The drawing under review shows one solid part. Ordinate dimensions are in mm from its lowest x, y, z. A direction names the side the tool comes from. Give positions to 0.01 mm unless a question says otherwise; leave off trailing zeros. Order: outer loops, then holes, each group sorted by start corner. A loop starts at its lowest first (then second) coordinate and runs counter-clockwise, first axis right, second up. Notation, with made-up numbers: (82, -37.5) -> (116, -37.5) arc R26 cw to (116, -6.5) -> close; hole circle Ø6 at (74.5, -23.75). An arc over 180 degrees is marked (long way). One line per item, written item: value. Start each with the question number.
1) Consider section A-A (x = 29.5). State the section outline as (y, z) points.
2) Consider section C-C (y = 54.5). State the section outline as (x, z) points, plus the area to 3 significant figures.
3) Wall thickness on line 1 along Y through (x, z) = (18.5, 11.75); line 2 along X through (y, z) = (67, 18.5): over which ranges is each line inside the solid? List them lowest first. Write a range as from..to.
4) Consider section B-B (z = 13). State the section outline as (x, y) points, plus the area to 3 significant figures.
5) The part is to be moulded in two halves that separate along X. For the marked faces 1, 2, 3 and 4, say which applies: released by +X, released by -X, zero draft, split by the parting line, or undercut.
6) For pin 1 (3 mm diameter, centred on y = 26.5, z = 14.5, fed in from -X), flat-tipped, find the tip position at first contact; note if it passes through.
7) Tool access review of the marked faces 5 and 6: name each direction out of +Z, -Z, +X, -X, +Y, -Y from which nothing blocks a thin tool from reaching the whole face with its end or side.
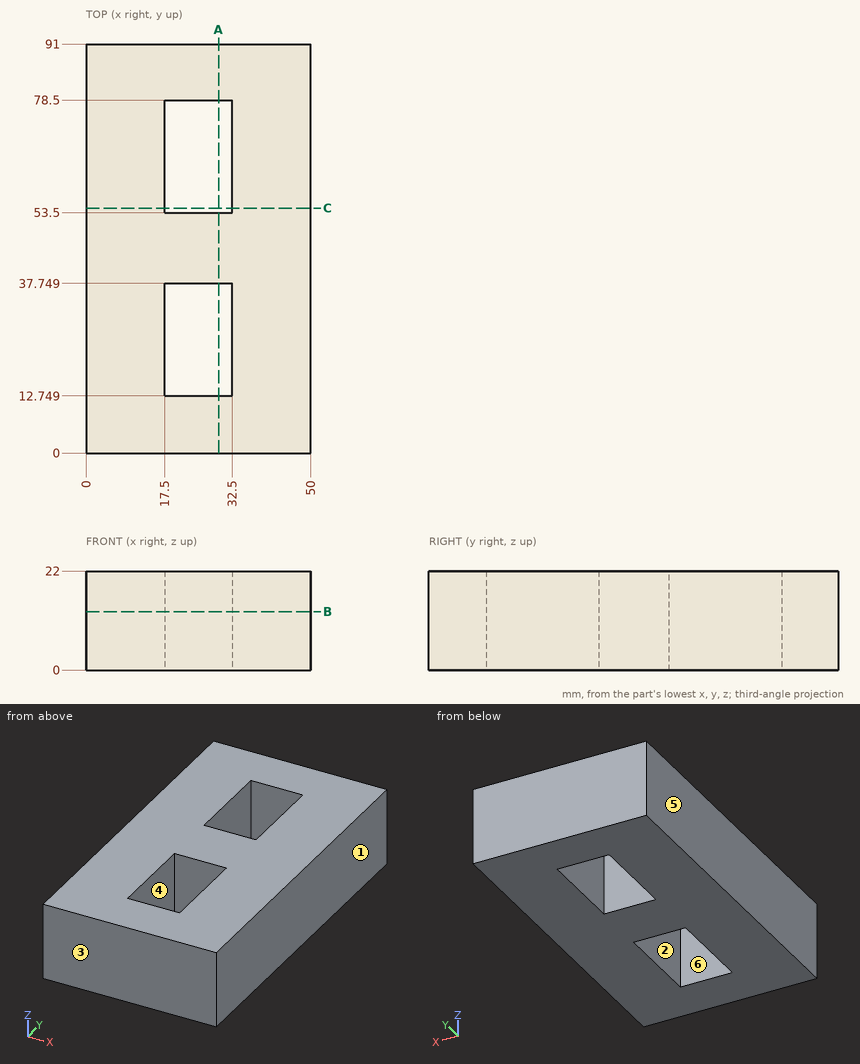
Checked values:
1. outline: (0, 0) -> (12.75, 0) -> (12.75, 22) -> (0, 22) -> close; (37.75, 0) -> (53.5, 0) -> (53.5, 22) -> (37.75, 22) -> close; (78.5, 0) -> (91, 0) -> (91, 22) -> (78.5, 22) -> close
2. outline: (0, 0) -> (17.5, 0) -> (17.5, 22) -> (0, 22) -> close; (32.5, 0) -> (50, 0) -> (50, 22) -> (32.5, 22) -> close
2. area: 770 mm^2
3. line 1: y = 0..12.75, 37.75..53.5, 78.5..91
3. line 2: x = 0..17.5, 32.5..50
4. outline: (0, 0) -> (50, 0) -> (50, 91) -> (0, 91) -> close; hole (17.5, 12.75) -> (32.5, 12.75) -> (32.5, 37.75) -> (17.5, 37.75) -> close; hole (17.5, 53.5) -> (32.5, 53.5) -> (32.5, 78.5) -> (17.5, 78.5) -> close
4. area: 3,800 mm^2
5. face 1: released by +X
5. face 2: undercut
5. face 3: zero draft
5. face 4: undercut
6. pin 1: stops at x = 0
7. face 5: +Z, -Z, -X, +Y, -Y
7. face 6: +Z, -Z
